Check sheet for the modelled part. Datum: model origin and axes. Units: mm. A direction names the side the tool comes from. Coordinates: 2 decimals unless noted, no trailing zeros. Loops run counter-clockwise (first coordinate to the right, second up) from the corner with the lowest first, then second, coordinate; pieces in that order, holes last. Notation, with made-up numbers: (58.25, -20) -> (103.25, -20) arc R30 ccw to (103.25, 9) -> close; hole circle Ø5 at (-8, -1.5). An arc over 180 degrees is marked (long way). Use CSV: the item, a comma, the result in double quotes. Start each with the question number.
1. Gauge pin test, flat end, axial feed: pin 1 (1.5 mm diameter, centred on x = -23.5, z = 32.5, fed in from +Y). Record the tip position at first contact, or that the pin passes through.
2. Sectioned sample at A-A, the plane z = 25.4. Record the cut outline in (x, y).
3. Sectioned sample at D-D, the plane x = -24. Record the cut outline in (y, z), and give its area (3 significant figures).
4. Release check for a two-part mould opening along X. For faces 1 (the face through (-30.8, 18.1, 50.8)), 2 (the face through (-17, 17.938, 25)), 3 (the face through (-6.764, 11, 25)) record: pulls with the +X half, pulls with the -X half, needs draft (parallel to the pull), parting line crosses it, or undercut.
5. Sectioned sample at C-C, the plane x = -48.5. Record the cut outline in (y, z).
6. Thickness scan on L1, parallel to X at y = 4.65, z = 25.4; L2, parallel to Y at x = -48, z = 10; L3, parallel to X at y = 8.25, z = 32. Record the ranges inside material, lowest first.
7. Sectioned sample at B-B, the plane y = 6.25. Record the cut outline in (x, z).
8. Set-up check for faces 4 (the face through (-44.468, 3.672, 34.055)), 5 (the face through (-51.087, 11, 25)): record each of +Z, -Z, +X, -X, +Y, -Y from which the full face is reachable in a straight line by a thin tool's end or side.
```python
from build123d import *

# Parameters (mm, degrees)
SKETCH1_W           = 47.498
SKETCH1_H           = 19.05
BOSS_EXTRUDE1_DEPTH = 50.8
SKETCH2_W           = 41.148
SKETCH2_H           = 12.7
CUT_EXTRUDE1_DEPTH  = 51.8
SKETCH5_R           = 14.224
CUT_EXTRUDE2_DEPTH  = 20.05


with BuildPart() as part:
    # Sketch1 → Boss-Extrude1 (new body)
    with BuildSketch(Plane.XY):
        with Locations((-30.51329874, 11.587546426)):
            Rectangle(SKETCH1_W, SKETCH1_H)
    extrude(amount=BOSS_EXTRUDE1_DEPTH)

    # Sketch2 → Cut-Extrude1 (cut, through all)
    with BuildSketch(Plane(origin=(0, 0, 0), x_dir=(-1, 0, 0), z_dir=(0, 0, -1))):
        with Locations((30.51329874, 11.587546426)):
            Rectangle(SKETCH2_W, SKETCH2_H)
    extrude(amount=-CUT_EXTRUDE1_DEPTH, mode=Mode.SUBTRACT)

    # Sketch5 → Cut-Extrude2 (cut, through all)
    with BuildSketch(Plane(origin=(0, 21.112546426, 0), x_dir=(1, 0, 0), z_dir=(0, 1, 0))):
        with Locations((-33.18029874, -25.4)):
            Circle(SKETCH5_R)
    extrude(amount=-CUT_EXTRUDE2_DEPTH, mode=Mode.SUBTRACT)


solid = part.part
```
Completed:
1,pin 1,"through"
2,outline,"(-54.26, 2.06) -> (-47.4, 2.06) -> (-47.4, 5.24) -> (-51.09, 5.24) -> (-51.09, 17.94) -> (-47.4, 17.94) -> (-47.4, 21.11) -> (-54.26, 21.11) -> close; (-18.96, 2.06) -> (-6.76, 2.06) -> (-6.76, 21.11) -> (-18.96, 21.11) -> (-18.96, 17.94) -> (-9.94, 17.94) -> (-9.94, 5.24) -> (-18.96, 5.24) -> close"
3,outline,"(2.06, 0) -> (5.24, 0) -> (5.24, 14.54) -> (2.06, 14.54) -> close; (2.06, 36.26) -> (5.24, 36.26) -> (5.24, 50.8) -> (2.06, 50.8) -> close; (17.94, 0) -> (21.11, 0) -> (21.11, 14.54) -> (17.94, 14.54) -> close; (17.94, 36.26) -> (21.11, 36.26) -> (21.11, 50.8) -> (17.94, 50.8) -> close"
3,area,"185 mm²"
4,face 1,"needs draft"
4,face 2,"undercut"
4,face 3,"pulls with the +X half"
5,outline,"(2.06, 0) -> (5.24, 0) -> (5.24, 50.8) -> (2.06, 50.8) -> close; (17.94, 0) -> (21.11, 0) -> (21.11, 50.8) -> (17.94, 50.8) -> close"
6,L1,"-54.26 to -47.4, -18.96 to -6.76"
6,L2,"2.06 to 5.24, 17.94 to 21.11"
6,L3,"-54.26 to -51.09, -9.94 to -6.76"
7,outline,"(-54.26, 0) -> (-51.09, 0) -> (-51.09, 50.8) -> (-54.26, 50.8) -> close; (-9.94, 0) -> (-6.76, 0) -> (-6.76, 50.8) -> (-9.94, 50.8) -> close"
8,face 4,"+Y, -Y"
8,face 5,"+Z, -Z"
